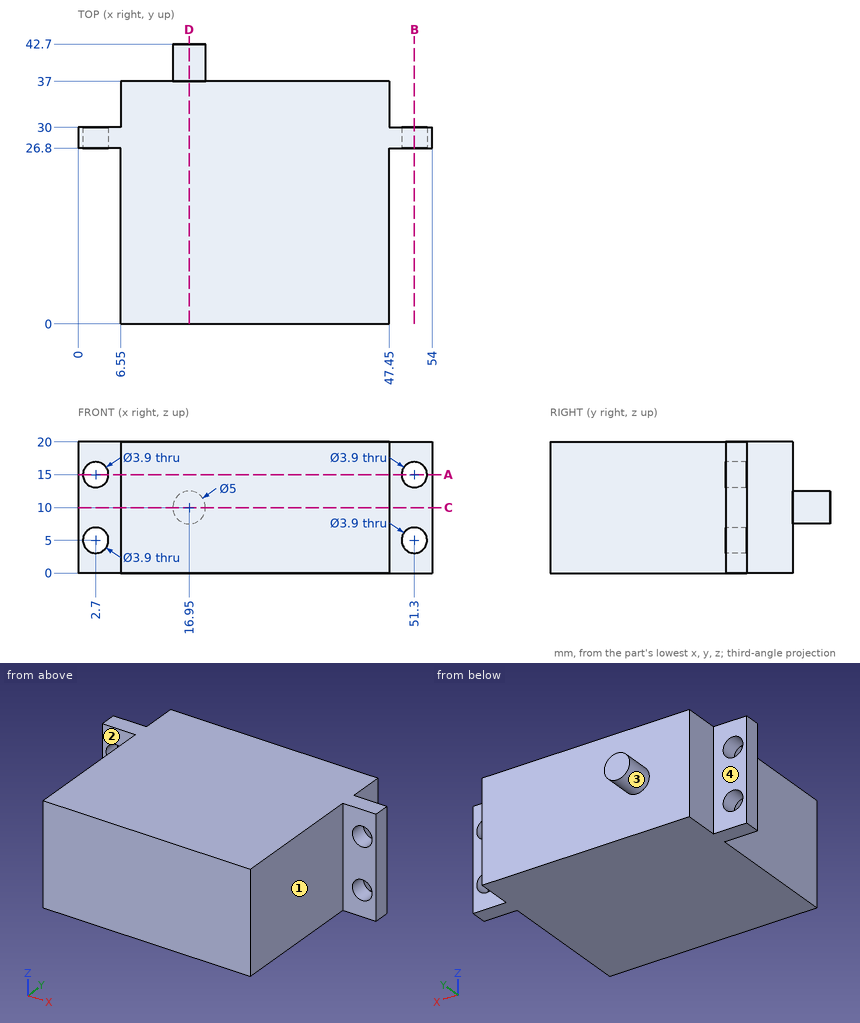
Verification items for this drawing (mm, ordinates from the low corner). A direction names the side the tool comes from. Give positions to 0.01 mm unless a question says otherwise; leave off trailing zeros. Loops run counter-clockwise (first coordinate to the right, second up) from the corner with the lowest first, then second, coordinate; pieces in that order, holes last. Notation, with made-up numbers: (42, 34) - (63, 34) arc R27 cw to (63, 57) - close; hole circle Ø9 at (45, 23). An arc over 180 degrees is marked (long way). Write item = value, one per line. Start each with the question number.
Q1. Depth check by flat-ended pin: P1, Ø3.5, axis at x = 3.5, z = 7, coming from the -Y side; P2, Ø3.5, axis at x = 2, z = 15, coming from the +Y side; P3, Ø2, axis at y = 33, z = 10, coming from the -X side; P4, Ø2.5, axis at x = 2.7, z = 5, coming from the +Y side. Enter the tip coordinate at first touch or a pass-through.
Q2. Cross-section at B-B, the plane x = 51.3. Enter the section's corners in (y, z), and give its area (3 significant figures).
Q3. Cross-section at A-A, the plane z = 15. Enter the section's corners in (x, y), and give its area (3 significant figures).
Q4. Thickness scan on line 1 (Z direction, x = 2.7, y = 27.7); line 2 (X direction, y = 29.35, z = 5); line 3 (Y direction, x = 24, z = 6). Record the ranges inside material, lowest first.
Q5. Cross-section at D-D, the plane x = 16.95. Enter the section's corners in (y, z).
Q6. Tool access check on the marked faces 1, 2, 3 and 4. Record the directions out of +Z, -Z, +X, -X, +Y, -Y that give a thin tool (end or side, any length) a straight path to the whole face; none if there is none.
Q7. Cross-section at C-C, the plane z = 10. Enter the section's corners in (x, y).
Answer key:
q1.P1 = 26.8
q1.P2 = 30
q1.P3 = 6.55
q1.P4 = through
q2.outline = (26.8, 0) - (30, 0) - (30, 3.05) - (26.8, 3.05) - close; (26.8, 6.95) - (30, 6.95) - (30, 13.05) - (26.8, 13.05) - close; (26.8, 16.95) - (30, 16.95) - (30, 20) - (26.8, 20) - close
q2.area = 39.0 mm^2
q3.outline = (0, 26.8) - (0.75, 26.8) - (0.75, 30) - (0, 30) - close; (4.65, 26.8) - (6.55, 26.8) - (6.55, 0) - (47.45, 0) - (47.45, 26.8) - (49.35, 26.8) - (49.35, 30) - (47.45, 30) - (47.45, 37) - (6.55, 37) - (6.55, 30) - (4.65, 30) - close; (53.25, 26.8) - (54, 26.8) - (54, 30) - (53.25, 30) - close
q3.area = 1,530 mm^2
q4.line_1 = 0 to 3.05, 6.95 to 13.05, 16.95 to 20
q4.line_2 = 0 to 0.75, 4.65 to 49.35, 53.25 to 54
q4.line_3 = 0 to 37
q5.outline = (0, 0) - (37, 0) - (37, 7.5) - (42.7, 7.5) - (42.7, 12.5) - (37, 12.5) - (37, 20) - (0, 20) - close
q6.face_1 = +Z, -Z, +X, -Y
q6.face_2 = +Z, -Z, -X, -Y
q6.face_3 = +Y
q6.face_4 = +Z, -Z, -X, +Y
q7.outline = (0, 26.8) - (6.55, 26.8) - (6.55, 0) - (47.45, 0) - (47.45, 26.8) - (54, 26.8) - (54, 30) - (47.45, 30) - (47.45, 37) - (19.45, 37) - (19.45, 42.7) - (14.45, 42.7) - (14.45, 37) - (6.55, 37) - (6.55, 30) - (0, 30) - close
